Input: part model. Units: mm. Frame: model coordinates. A direction names the side the tool comes from. Give positions to 0.01 mm unless a question says otherwise; leave off trailing zeros. Loops run counter-clockwise (first coordinate to the right, second up) from the corner with the lowest first, then second, coordinate; pieces in that order, holes last. Notation, with made-up numbers: M 47.25,27.5 L 58.25,27.5 A26 cw 58.25,56.5 Z; hole C -3.5,-5.75 d5. An arc over 180 degrees is marked long. One line per item, written item: value. Start each with the question number.
(1) Section B-B on z = 924.5. Output: boundary loops of the cut face in (x, y), plus the area to 3 significant figures.
(2) Ray query, line 1 along Z through (x, y) = (-20, 48); line 2 along Y through (x, z) = (-25, 1286); line 3 along X through (y, z) = (41, 310). Return the intervals inside material, ascending. Write a range as from..to.
(3) Access query for faces 1 (the flat face through (0, 25, 986)), 2 (the flat face through (-25, 45, 986)). Directions: +Z, -Z, +X, -X, +Y, -Y. A direction counts if a zero-diameter tool reaches every point of the face in a straight line with its end or side. Return the directions, or none.
(4) Section A-A on y = 31.5. Output: boundary loops of the cut face in (x, z).
(5) Pull-direction query (Y, two-part tool) for faces 3 (the flat face through (-50, 25, 986)), 4 (the flat face through (-25, 0, 986)), 5 (the flat face through (-5, 25, 986)); classes: released by +Y, released by -Y, zero draft, split by the parting line, or undercut.
(6) Pin query (flat end, axial travel): P1, Ø9.5, axis at x = -20, z = 550, coming from the -Y side. Return the tip coordinate at first contact, or that it passes through.
Autodesk Inventor part; units mm, degrees
ref_plane "YZ Plane" through (0, 0, 0) normal (1, 0, 0) x (0, 1, 0)
ref_plane "XZ Plane" through (0, 0, 0) normal (0, 1, 0) x (-1, 0, 0)
ref_plane "XY Plane" through (0, 0, 0) normal (0, 0, 1) x (1, 0, 0)
sketch "Sketch1" plane through (0, 0, 0) normal (0, 0, 1) x (1, 0, 0)
  line L0 (-8, 0) -> (-42, 0)
  line L1 (-50, 8) -> (-50, 42)
  line L2 (-42, 50) -> (-8, 50)
  line L3 (0, 42) -> (0, 8)
  arc A0 (-42, 50) -> (-50, 42) centre (-42, 42) ccw
  arc A1 (0, 42) -> (-8, 50) centre (-8, 42) ccw
  arc A2 (-8, 0) -> (0, 8) centre (-8, 8) ccw
  arc A3 (-50, 8) -> (-42, 0) centre (-42, 8) ccw
  line L4 (-45, 42) -> (-45, 8)
  arc A4 (-45, 8) -> (-42, 5) centre (-42, 8) ccw
  line L5 (-42, 5) -> (-8, 5)
  arc A5 (-8, 5) -> (-5, 8) centre (-8, 8) ccw
  line L6 (-5, 8) -> (-5, 42)
  arc A6 (-5, 42) -> (-8, 45) centre (-8, 42) ccw
  line L7 (-8, 45) -> (-42, 45)
  arc A7 (-42, 45) -> (-45, 42) centre (-42, 42) ccw
  point P0 (0, 0)
  point P1 (-50, 50)
  point P2 (-50, 0)
  point P3 (0, 50)
  dimension "d0" = 50
  dimension "d1" = 50
  dimension "d2" = 8
  dimension "d3" = 5
extrude "Extrusion1" add sketch "Sketch1" along normal blind 2000
sketch "Sketch2" plane through (-42, 50, 0) normal (0, 1, 0) x (1, 0, 0)
  line L0 (0, 0) -> (34, 0)
  line L1 (34, 0) -> (34, -54.5049)
  line L2 (34, 0) -> (34, -2000)
  circle A0 centre (22, -100) radius 3
  point P0 (42, 0)
  point P1 (22, -550)
  point P2 (22, -1000)
  point P3 (22, -1450)
  dimension "d6" = 20
  dimension "d7" = 100
  dimension "d10" = 450
  dimension "d22" = 6
extrude "Extrusion2" cut sketch "Sketch2" against normal through all
pattern_linear "Rectangular Pattern1" count 2 spacing 450 along (0, 0, 1) of "Extrusion2"
ref_plane "Work Plane1" through (-20, 50, 550) normal (1, 0, 0) x (0, -1, 0)
properties part number "50x50x5"
Output values:
1. outline: M -50,8 A8 ccw -42,0 L -8,0 A8 ccw 0,8 L 0,42 A8 ccw -8,50 L -42,50 A8 ccw -50,42 Z; hole M -45,8 A3 ccw -42,5 L -8,5 A3 ccw -5,8 L -5,42 A3 ccw -8,45 L -42,45 A3 ccw -45,42 Z
1. area: 853 mm²
2. line 1: z = 0..97, 103..547, 553..2000
2. line 2: y = 0..5, 45..50
2. line 3: x = -50..-45, -5..0
3. face 1: +Z, -Z, +X, +Y, -Y
3. face 2: +Z, -Z
4. outline: M -50,0 L -45,0 L -45,2000 L -50,2000 Z; M -5,0 L 0,0 L 0,2000 L -5,2000 Z
5. face 3: zero draft
5. face 4: released by -Y
5. face 5: undercut
6. P1: stops at y = 0
